from build123d import *

# Parameters (mm, degrees)
CUT_EXTRUDE1_DEPTH = 2.5
FILLET4_R          = 1
FILLET5_R          = 1
CUT_EXTRUDE3_DEPTH = 2.5


with BuildPart() as part:
    # Sketch1 → Revolve1 (revolve)
    with BuildSketch(Plane.XY, mode=Mode.PRIVATE) as revolve1_sk:
        Polygon((111.690273615, 0), (111.690273615, 12.5), (17.690273615, 12.5), (17.690273615, 13), (-54.309726385, 13), (-54.309726385, 12.5), (-88.409726385, 12.5), (-88.409726385, 0), align=None)
    revolve(revolve1_sk.sketch.rotate(Axis((-88.409726385, 0, 0), (1, 0, 0)), 180), axis=Axis((-88.409726385, 0, 0), (1, 0, 0)))

    # Sketch2 → Cut-Extrude1 (cut)
    with BuildSketch(Plane(origin=(0, 12.5, 0), x_dir=(1, 0, 0), z_dir=(0, 1, 0))):
        with BuildLine():
            Line((26.390273615, 2.5), (49.390273615, 2.5))
            ThreePointArc((49.390273615, 2.5), (51.890273615, 0), (49.390273615, -2.5))
            Line((49.390273615, -2.5), (26.390273615, -2.5))
            ThreePointArc((26.390273615, -2.5), (23.890273615, 0), (26.390273615, 2.5))
        make_face()
    extrude(amount=-CUT_EXTRUDE1_DEPTH, mode=Mode.SUBTRACT)

    # Fillet4
    fillet4_edges = [part.edges().sort_by_distance(p)[0] for p in [
        (111.690273615, 12.5, 0),
    ]]
    fillet(fillet4_edges, radius=FILLET4_R)

    # Fillet5
    fillet5_edges = [part.edges().sort_by_distance(p)[0] for p in [
        (-88.409726385, 12.5, 0),
    ]]
    fillet(fillet5_edges, radius=FILLET5_R)

    # Sketch3 → Cut-Extrude3 (cut)
    with BuildSketch(Plane(origin=(0, 13, 0), x_dir=(1, 0, 0), z_dir=(0, 1, 0))):
        with BuildLine():
            Line((-29.809726385, 2.5), (-6.809726385, 2.5))
            ThreePointArc((-6.809726385, 2.5), (-4.309726385, 0), (-6.809726385, -2.5))
            Line((-6.809726385, -2.5), (-29.809726385, -2.5))
            ThreePointArc((-29.809726385, -2.5), (-32.309726385, 0), (-29.809726385, 2.5))
        make_face()
    extrude(amount=-CUT_EXTRUDE3_DEPTH, mode=Mode.SUBTRACT)


solid = part.part
The listing builds one solid part. Answer for the finished solid, in the listing's coordinates (mm). A direction names the side the tool comes from. Round coordinates to 2 decimals unless told otherwise and drop trailing zeros. Order: outer loops, then holes, each group sorted by start corner. A loop starts at its lowest first (then second) coordinate and runs counter-clockwise, first axis right, second up. Notation, with made-up numbers: M 53,-30.5 L 97,-30.5 A30 ccw 97,-0.5 Z; hole C -12.5,13 d2. An arc over 180 degrees is marked long. Answer in a Markdown table with one row per item. Add a question column.
1) The part is cut by section A-A on z = 0. Determine the outline of the cut face in (x, y).
2) Determine the mould class of faces 1 (the face through (-54.31, 6.8, -10.7)), 2 (the face through (-71.091, -11.923, -3.755)), 3 (the face through (38, 10, 0)) for opening direction X: pulls with the +X half, pulls with the -X half, needs draft (parallel to the pull), parting line crosses it, or undercut.
3) The part is cut by section C-C on x = -43. Determine the outline of the cut face in (y, z), plus the area to 3 significant figures.
4) Flat-ended cylindrical pins translate along their axes: pin 1 Ø1.5 at (x, z) = (22, 5.5) entering from -Y; pin 2 Ø2.5 at (x, z) = (34.5, -0.5) entering from +Y; pin 3 Ø1.5 at (x, z) = (8, -2.5) entering from +Y. Find the tip coordinate at first contact, or state that the pin passes through.
5) The part is cut by section D-D on x = 63. Determine the outline of the cut face in (y, z), plus the area to 3 significant figures.
6) Which of the six approach directions +Z, -Z, +X, -X, +Y, -Y give full straight-line access (tool end or side, diameter ignored) to faces 4 (the face through (111.69, 0, 0)), 5 (the face through (-18, 10.5, 0)), 6 (the face through (17.69, -6.8, -10.7))?
7) Consider line 1 along Z through (x, y) = (32.5, -0.25); line 2 along Y through (x, z) = (-6, -6); line 3 along Y through (x, z) = (-59, 1). Determine where each line is inside the solid, lowest interval first. Write a range as from..to.
8) The part is cut by section B-B on y = 0. Determine the outline of the cut face in (x, z), plus the area to 3 significant figures.
Findings below:
| question | item | result |
|---|---|---|
| 1 | outline | M -88.41,-11.5 A1 ccw -87.41,-12.5 L -54.31,-12.5 L -54.31,-13 L 17.69,-13 L 17.69,-12.5 L 110.69,-12.5 A1 ccw 111.69,-11.5 L 111.69,11.5 A1 ccw 110.69,12.5 L 51.89,12.5 L 51.89,10 L 23.89,10 L 23.89,12.5 L 17.69,12.5 L 17.69,13 L -4.31,13 L -4.31,10.5 L -32.31,10.5 L -32.31,13 L -54.31,13 L -54.31,12.5 L -87.41,12.5 A1 ccw -88.41,11.5 Z |
| 2 | face 1 | pulls with the -X half |
| 2 | face 2 | needs draft |
| 2 | face 3 | undercut |
| 3 | outline | C 0,0 d26 |
| 3 | area | 531 mm² |
| 4 | pin 1 | stops at y = -11.56 |
| 4 | pin 2 | stops at y = 10 |
| 4 | pin 3 | stops at y = 12.88 |
| 5 | outline | C 0,0 d25 |
| 5 | area | 491 mm² |
| 6 | face 4 | +Z, -Z, +X, +Y, -Y |
| 6 | face 5 | +Y |
| 6 | face 6 | +X |
| 7 | line 1 | z = -12.5..12.5 |
| 7 | line 2 | y = -11.53..11.53 |
| 7 | line 3 | y = -12.46..12.46 |
| 8 | outline | M -88.41,-11.5 A1 ccw -87.41,-12.5 L -54.31,-12.5 L -54.31,-13 L 17.69,-13 L 17.69,-12.5 L 110.69,-12.5 A1 ccw 111.69,-11.5 L 111.69,11.5 A1 ccw 110.69,12.5 L 17.69,12.5 L 17.69,13 L -54.31,13 L -54.31,12.5 L -87.41,12.5 A1 ccw -88.41,11.5 Z |
| 8 | area | 5,070 mm² |
